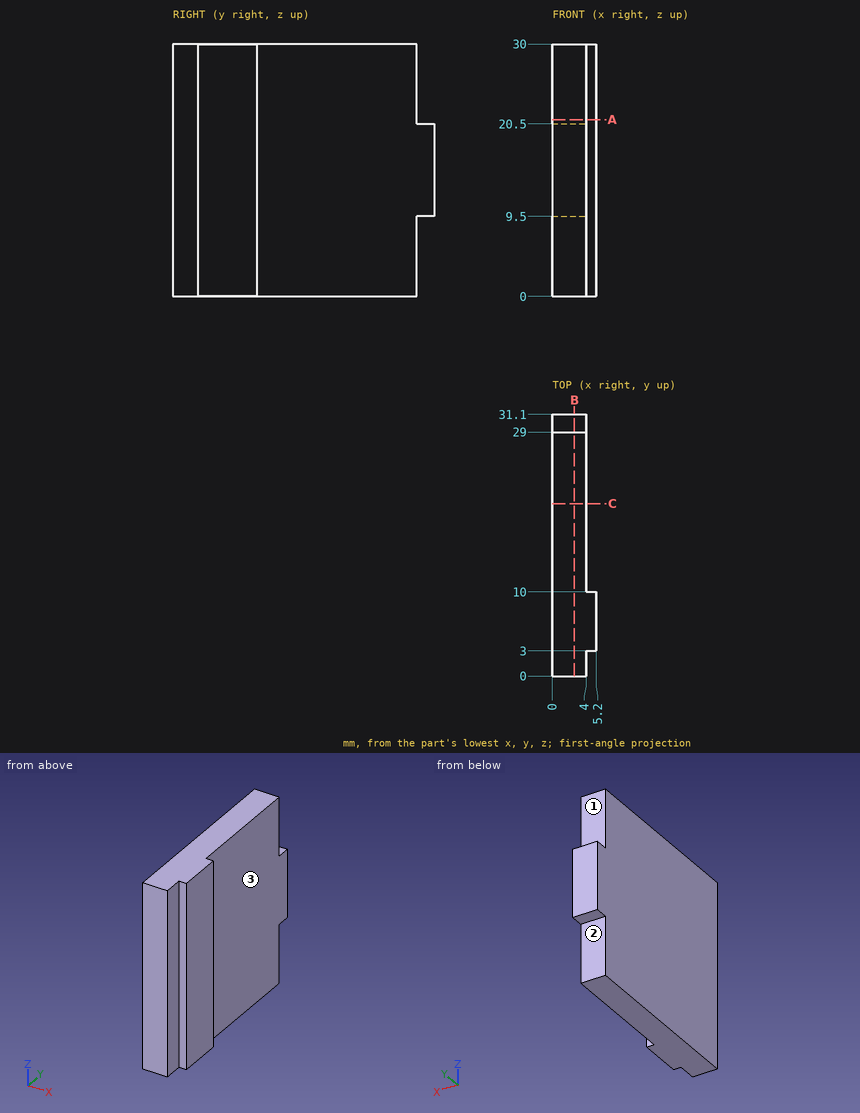
Here's the drawing with two shaded views (mm, measured from the low corner). I have some questions. A direction names the side the tool comes from. Coordinates: 2 decimals unless noted, no trailing zeros. Write each loop counter-clockwise with the first axis right and the second up, starting at its lowest first coordinate (ties: lowest second). Pieces come first, ordered by that corner, then holes. Notation, with made-up numbers: M 30.25,6 L 42.25,6 A27 cw 42.25,29 Z; hole C 62.25,4 d5. An arc over 180 degrees is marked long. Write item = value, one per line. Start each with the question number.
Q1. On a 3-axis mill with a long thin cutter (end or side, diameter ignored), from which of +Z, -Z, +X, -X, +Y, -Y can I reach the whole of each face in a straight line? I mean the marked faces 1, 2 and 3. Say none if no direction works.
Q2. If I drill on L1, parallel to X at y = 21.5, z = 19; L2, parallel to Y at x = 1.55, z = 27.75; L3, parallel to Y at x = 4.4, z = 8.25, over which ranges is the centre line in solid material (lowest first)? Write a range as [from, to].
Q3. I'm going to push flat-ended pins straight in: pin 1 (3 mm diameter, centred on x = 2.5, z = 26.5, fed in from +Y); pin 2 (4 mm diameter, centred on y = 14.5, z = 23.5, fed in from +X); pin 3 (0.6 mm diameter, centred on x = 1.5, y = 30, fed in from -Z). Where does each tip first touch, or does it pass through?
Q4. If we section it at C-C, the plane y = 20.5: Write out the boundary of the cut face in (x, z), then the cut area to 3 significant figures.
Q5. If we section it at B-B, the plane x = 2.6: Write out the boundary of the cut face in (y, z).
Q6. If we section it at A-A, the plane z = 21: Write out the boundary of the cut face in (x, y), then the cut area to 3 significant figures.
Check sheet entries:
q1.face_1 = +Z, +X, -X, +Y
q1.face_2 = -Z, +X, -X, +Y
q1.face_3 = +Z, -Z, +X, +Y
q2.L1 = [0, 4]
q2.L2 = [0, 29]
q2.L3 = [3, 10]
q3.pin_1 = 29
q3.pin_2 = 4
q3.pin_3 = 9.5
q4.outline = M 0,0 L 4,0 L 4,30 L 0,30 Z
q4.area = 120 mm²
q5.outline = M 0,0 L 29,0 L 29,9.5 L 31.1,9.5 L 31.1,20.5 L 29,20.5 L 29,30 L 0,30 Z
q6.outline = M 0,0 L 4,0 L 4,3 L 5.2,3 L 5.2,10 L 4,10 L 4,29 L 0,29 Z
q6.area = 124 mm²
